Read the model definition and answer for the solid it produces. Units are mm, in the model's axes. A direction names the side the tool comes from. Give positions to 0.01 mm unless a question says otherwise; leave off trailing zeros. Order: outer loops, then holes, each group sorted by start corner. A loop starts at its lowest first (then second) coordinate and runs counter-clockwise, first axis right, second up. Notation, with made-up numbers: (-3.5, 68) - (45.5, 68) arc R19 ccw to (45.5, 75) - close; hole circle Ø9 at (54.25, -11.5). An arc over 180 degrees is marked (long way). Return JSON: item names as keys, results as strings.
```python
from build123d import *

# Parameters (mm, degrees)
SKETCH2_W           = 50
SKETCH2_H           = 25
SKETCH2_R           = 3.175
BOSS_EXTRUDE1_DEPTH = 3.175
SKETCH11_W          = 18
SKETCH11_H          = 25
BOSS_EXTRUDE4_DEPTH = 3.175
SKETCH12_W          = 44.125
SKETCH12_H          = 17.175
BOSS_EXTRUDE5_DEPTH = 7.275
SKETCH13_W          = 45.360945172
SKETCH13_H          = 22.695099396
CUT_EXTRUDE1_DEPTH  = 1.6
CUT_EXTRUDE2_DEPTH  = 76.525368255
BOSS_EXTRUDE6_DEPTH = 3.175
BOSS_EXTRUDE7_DEPTH = 3.175
FILLET7_R           = 1.5
SKETCH17_W          = 2.5
SKETCH17_H          = 7.62
SKETCH17_H_2        = 6
CUT_EXTRUDE3_DEPTH  = 14


with BuildPart() as part:
    # Sketch2 → Boss-Extrude1 (new body)
    with BuildSketch(Plane(origin=(0, 0, 0), x_dir=(1, 0, 0), z_dir=(0, 1, 0))):
        Rectangle(SKETCH2_W, SKETCH2_H)
        with Locations(Location((-12.7, 0, 0), (0, 0, 270))):
            Circle(SKETCH2_R, mode=Mode.SUBTRACT)
        with Locations(Location((12.7, 0, 0), (0, 0, 270))):
            Circle(SKETCH2_R, mode=Mode.SUBTRACT)
    extrude(amount=BOSS_EXTRUDE1_DEPTH)

    # Sketch11 → Boss-Extrude4 (add)
    with BuildSketch(Plane(origin=(0, 0, 0), x_dir=(1, 0, 0), z_dir=(0, 1, 0))):
        with Locations((-34, 0)):
            Rectangle(SKETCH11_W, SKETCH11_H)
    extrude(amount=BOSS_EXTRUDE4_DEPTH)

    # Sketch12 → Boss-Extrude5 (add)
    with BuildSketch(Plane.ZY.offset(43)):
        with Locations((9.5625, 8.5875)):
            Rectangle(SKETCH12_W, SKETCH12_H)
    extrude(amount=-BOSS_EXTRUDE5_DEPTH)

    # Sketch13 → Cut-Extrude1 (cut)
    with BuildSketch(Plane.ZY.offset(43)):
        with Locations((5.769527414, 14.522549698)):
            Rectangle(SKETCH13_W, SKETCH13_H)
    extrude(amount=-CUT_EXTRUDE1_DEPTH, mode=Mode.SUBTRACT)

    # Sketch14 → Cut-Extrude2 (cut, through all)
    with BuildSketch(Plane.ZY.offset(41.4)):
        with BuildLine():
            Line((6.45, 8.675), (0.442633339, 8.675))
            ThreePointArc((0.442633339, 8.675), (-1.057366661, 10.175), (0.442633339, 11.675))
            Line((0.442633339, 11.675), (6.45, 11.675))
            ThreePointArc((6.45, 11.675), (7.95, 10.175), (6.45, 8.675))
        make_face()
    extrude(amount=-CUT_EXTRUDE2_DEPTH, mode=Mode.SUBTRACT)

    # Sketch15 → Boss-Extrude6 (add)
    with BuildSketch(Plane(origin=(0, 0, -12.5), x_dir=(-1, 0, 0), z_dir=(0, 0, -1))):
        Polygon((35.725, 17.175), (24.225, 3.175), (35.725, 3.175), align=None)
    boss_extrude6 = extrude(amount=-BOSS_EXTRUDE6_DEPTH)

    # Mirror1: Boss-Extrude6 across plane
    add(boss_extrude6.mirror(Plane.XY))

    # Sketch16 → Boss-Extrude7 (add)
    with BuildSketch(Plane.XZ):
        Polygon((-35.725, 12.5), (-28.225, 12.5), (-35.725, 22.5), align=None)
    extrude(amount=-BOSS_EXTRUDE7_DEPTH)

    # Fillet7
    fillet7_edges = [part.edges().sort_by_distance(p)[0] for p in [
        (-29.975, 10.175, 12.5),
        (-29.975, 10.175, -12.5),
        (0.3875, 3.175, 12.5),
        (25, 1.5875, 12.5),
        (25, 3.175, 0),
        (25, 1.5875, -12.5),
        (0.3875, 3.175, -12.5),
        (-35.725, 10.175, -9.325),
        (-29.975, 3.175, -9.325),
        (-29.975, 3.175, 9.325),
        (-35.725, 10.175, 9.325),
        (-35.725, 3.175, 0),
        (-31.975, 3.175, 17.5),
        (-24.225, 3.175, -10.9125),
        (-24.225, 3.175, 10.9125),
        (-35.725, 8.5875, 31.625),
    ]]
    fillet(fillet7_edges, radius=FILLET7_R)

    # Sketch17 → Cut-Extrude3 (cut)
    with BuildSketch(Plane(origin=(0, 17.175, 0), x_dir=(1, 0, 0), z_dir=(0, 1, 0))):
        with Locations((-40.15, -24.64)):
            Rectangle(SKETCH17_W, SKETCH17_H)
        with Locations((-40.15, 1.55)):
            Rectangle(SKETCH17_W, SKETCH17_H_2)
    extrude(amount=-CUT_EXTRUDE3_DEPTH, mode=Mode.SUBTRACT)


solid = part.part
```
Q1. For faces 4 (the flat face through (-39, 11.675, 3)), 5 (the flat face through (-40, 14, 1.45)), 6 (the cylindrical face through (-35.3, 11.01, -8.87)), determine the directions among +Z, -Z, +X, -X, +Y, -Y from which every point of the face is accessible in a straight line to the end or side of a thin tool.
Values:
{"face 4": "+X, -X", "face 5": "-X, +Y", "face 6": "+X, +Y"}
Q2. Given pin 1 (6.5 mm diameter, centred on x = -18.5, z = 2, fed in from +Y) (3 decimals); pin 2 (3 mm diameter, centred on y = 10.5, z = 4.5, fed in from +X) (3 decimals); pin 3 (6 mm diameter, centred on x = -6, z = 0, fed in from -Y); pin 4 (5 mm diameter, centred on x = 12.7, z = 0, fed in from +Y), each flat-ended and moving along its own axis, determine where each tip first touches the part or whether it passes through.
Values:
{"pin 1": "stops at y = 3.175", "pin 2": "stops at x = -35.725", "pin 3": "stops at y = 0", "pin 4": "passes through"}
Q3. A cutting plane is placed at A-A (x = 12.7). Write down the section's boundary in (y, z) (3 decimals).
Values:
{"outline": "(0, -12.5) - (1.675, -12.5) arc R1.5 ccw to (3.175, -11) - (3.175, -3.175) - (0, -3.175) - close; (0, 3.175) - (3.175, 3.175) - (3.175, 11) arc R1.5 ccw to (1.675, 12.5) - (0, 12.5) - close"}
Q4. A cutting plane is placed at B-B (y = 1). Write down the section's boundary in (x, z) (3 decimals), and give its area (3 significant figures).
Values:
{"outline": "(-43, -12.5) - (23.5, -12.5) arc R1.5 ccw to (25, -11) - (25, 11) arc R1.5 ccw to (23.5, 12.5) - (-28.225, 12.5) - (-35.725, 22.5) - (-35.725, 30.125) arc R1.5 ccw to (-37.225, 31.625) - (-43, 31.625) - close; hole circle Ø6.35 at (-12.7, 0); hole circle Ø6.35 at (12.7, 0)", "area": "1,810 mm²"}
Q5. Determine the mould class of faces 1 (the flat face through (-40, 8, 31.625)), 2 (the flat face through (-38.9, 10, -2)), 3 (the flat face through (-9, 0, 0)) for opening direction Z: released by +Z, released by -Z, zero draft, split by the parting line, or undercut.
Values:
{"face 1": "released by +Z", "face 2": "undercut", "face 3": "zero draft"}
Q6. Consider L1, parallel to X at y = 1.5, z = 0 (3 decimals); L2, parallel to Z at x = -37, y = 12.5; L3, parallel to X at y = 6.25, z = 24 (3 decimals). Determine where each line is inside the solid, lowest interval first.
Values:
{"L1": "x = -43 to -15.875, -9.525 to 9.525, 15.875 to 25", "L2": "z = -12.5 to 31.61", "L3": "x = -38.9 to -35.725"}
Q7. A cutting plane is placed at C-C (x = -7). Write down the section's boundary in (y, z) (3 decimals), and give its area (3 significant figures).
Values:
{"outline": "(0, -12.5) - (1.675, -12.5) arc R1.5 ccw to (3.175, -11) - (3.175, 11) arc R1.5 ccw to (1.675, 12.5) - (0, 12.5) - close", "area": "78.4 mm²"}
